For this review, take the finished solid that the model builds, in its own axes (mm). A direction names the side the tool comes from. Coordinates: 2 decimals unless noted, no trailing zeros. Order: outer loops, then holes, each group sorted by start corner. A loop starts at its lowest first (then second) coordinate and runs counter-clockwise, first axis right, second up.
from build123d import *

# Parameters (mm, degrees)
SKETCH1_W           = 25.4
SKETCH1_H           = 17.78
BOSS_EXTRUDE1_DEPTH = 2
SKETCH2_R           = 1.27
CUT_EXTRUDE1_DEPTH  = 3
SKETCH3_W           = 5.5
SKETCH3_H           = 6
BOSS_EXTRUDE2_DEPTH = 2.9
FILLET1_R           = 2.54


with BuildPart() as part:
    # Sketch1 → Boss-Extrude1 (new body)
    with BuildSketch(Plane(origin=(0, 0, 0), x_dir=(1, 0, 0), z_dir=(0, 1, 0))):
        with Locations((12.7, 8.89)):
            Rectangle(SKETCH1_W, SKETCH1_H)
    extrude(amount=BOSS_EXTRUDE1_DEPTH)

    # Sketch2 → Cut-Extrude1 (cut, through all)
    with BuildSketch(Plane(origin=(0, 2, 0), x_dir=(1, 0, 0), z_dir=(0, 1, 0))):
        with Locations((2.54, 15.24)):
            Circle(SKETCH2_R)
        with Locations((22.86, 15.24)):
            Circle(SKETCH2_R)
        with Locations((22.86, 2.54)):
            Circle(SKETCH2_R)
        with Locations((2.54, 2.54)):
            Circle(SKETCH2_R)
    extrude(amount=-CUT_EXTRUDE1_DEPTH, mode=Mode.SUBTRACT)

    # Sketch3 → Boss-Extrude2 (add)
    with BuildSketch(Plane(origin=(0, 2, 0), x_dir=(1, 0, 0), z_dir=(0, 1, 0))):
        with Locations((22.65, 8.89)):
            Rectangle(SKETCH3_W, SKETCH3_H)
        with Locations((2.75, 8.89)):
            Rectangle(SKETCH3_W, SKETCH3_H)
    extrude(amount=BOSS_EXTRUDE2_DEPTH)

    # Fillet1
    fillet1_edges = [part.edges().sort_by_distance(p)[0] for p in [
        (0, 1, -17.78),
        (25.4, 1, -17.78),
        (25.4, 1, 0),
        (0, 1, 0),
    ]]
    fillet(fillet1_edges, radius=FILLET1_R)


solid = part.part
1. Take a section at A-A, the plane x = 23.75. Give the boundary of the cut face in (y, z), plus the area to 3 significant figures.
Answer below:
outline: (0, -17.62) - (2, -17.62) - (2, -16.15) - (0, -16.15) - close; (0, -14.33) - (2, -14.33) - (2, -11.89) - (4.9, -11.89) - (4.9, -5.89) - (2, -5.89) - (2, -3.45) - (0, -3.45) - close; (0, -1.63) - (2, -1.63) - (2, -0.16) - (0, -0.16) - close
area: 45.1 mm2
2. To check wall thickness, follow L1, parallel to Z at x = 22.86, y = 1.5; L2, parallel to X at y = 1, z = -15.24; L3, parallel to Y at x = 21.5, z = -1.25. State the ranges of each line that lie inside material, in increasing order.
Answer below:
L1: z = -17.78 to -16.51, -13.97 to -3.81, -1.27 to 0
L2: x = 0 to 1.27, 3.81 to 21.59, 24.13 to 25.4
L3: y = 0 to 2
3. Machinability: for faces 4 (the face through (23, 3, -5.89)), 5 (the face through (19.9, 3, -9)), 6 (the face through (3, 3, -11.89)), 7 (the face through (3, 4.9, -9)), which of the approach directions +Z, -Z, +X, -X, +Y, -Y give a long, thin tool a straight path to every point of the face, cutting with its end or side? Answer none if there is none.
Answer below:
face 4: +Z, +X, -X, +Y
face 5: +Z, -Z, +Y
face 6: -Z, +X, -X, +Y
face 7: +Z, -Z, +X, -X, +Y
4. Take a section at D-D, the plane x = 4.5. Give the boundary of the cut face in (y, z), plus the area to 3 significant figures.
Answer below:
outline: (0, -17.78) - (2, -17.78) - (2, -11.89) - (4.9, -11.89) - (4.9, -5.89) - (2, -5.89) - (2, 0) - (0, 0) - close
area: 53.0 mm2
5. Take a section at B-B, the plane y = 4.05. Give the boundary of the cut face in (x, z).
Answer below:
outline: (0, -11.89) - (5.5, -11.89) - (5.5, -5.89) - (0, -5.89) - close; (19.9, -11.89) - (25.4, -11.89) - (25.4, -5.89) - (19.9, -5.89) - close
6. The part is to be moulded in two halves that separate along Z. For faces 1 (the face through (23, 3, -11.89)), 2 (the face through (24.636, 1.014, -0.724)), 3 (the face through (22.7, 1, -16.5)), say which applies: +Z half, -Z half, draft (parallel to the pull), parting line (faces both ways), or undercut.
Answer below:
face 1: -Z half
face 2: +Z half
face 3: undercut
7. Clearance check with flat-ended pins moving along their axes: pin 1 Ø1.5 at (x, y) = (22.5, 4) entering from -Z; pin 2 Ø3 at (x, z) = (9, -4) entering from +Y; pin 3 Ø0.9 at (x, y) = (22.5, 4) entering from +Z. State where each tip first meets the part, or that it passes through.
Answer below:
pin 1: stops at z = -11.89
pin 2: stops at y = 2
pin 3: stops at z = -5.89
8. Take a section at C-C, the plane z = -7.25. Give the boundary of the cut face in (x, y).
Answer below:
outline: (0, 0) - (25.4, 0) - (25.4, 4.9) - (19.9, 4.9) - (19.9, 2) - (5.5, 2) - (5.5, 4.9) - (0, 4.9) - close
